Read the model definition and answer for the solid it produces. Units are mm, in the model's axes. Face numbers are marked on the shaded views. A direction names the side the tool comes from. Coordinates: 2 decimals unless noted, no trailing zeros. Write each loop counter-clockwise with the first axis right and the second up, starting at its lowest first coordinate (ties: lowest second). Pieces come first, ordered by that corner, then holes. Notation, with made-up numbers: (68, 49) -> (104, 49) arc R13 cw to (104, 54) -> close; hole circle Ø10 at (25.25, 27). An arc over 180 degrees is marked (long way). One line per item, written item: value. Start each with the question number.
from build123d import *

# Parameters (mm, degrees)
ESQUISSE1_R             = 9
ESQUISSE1_R_2           = 5.25
BOSS_EXTRU_1_DEPTH      = 13
ENL_V_MAT_EXTRU_1_DEPTH = 7
CHANFREIN1_SIZE         = 1


with BuildPart() as part:
    # Esquisse1 → Boss.-Extru.1 (new body)
    with BuildSketch(Plane.XY):
        with Locations(Location((0, 0, 0), (0, 0, 180))):
            Circle(ESQUISSE1_R)
        with Locations(Location((0, 0, 0), (0, 0, 180))):
            Circle(ESQUISSE1_R_2, mode=Mode.SUBTRACT)
    extrude(amount=BOSS_EXTRU_1_DEPTH)

    # Esquisse2 → Enlèv. mat.-Extru.1 (cut)
    with BuildSketch(Plane.XY.offset(13)):
        Polygon((3.75277675, 6.5), (-3.75277675, 6.5), (-7.505553499, 0), (-3.75277675, -6.5), (3.75277675, -6.5), (7.505553499, 0), align=None)
    extrude(amount=-ENL_V_MAT_EXTRU_1_DEPTH, mode=Mode.SUBTRACT)

    # Chanfrein1
    chanfrein1_edges = [part.edges().sort_by_distance(p)[0] for p in [
        (9, 0, 13),
    ]]
    chamfer(chanfrein1_edges, length=CHANFREIN1_SIZE)


solid = part.part
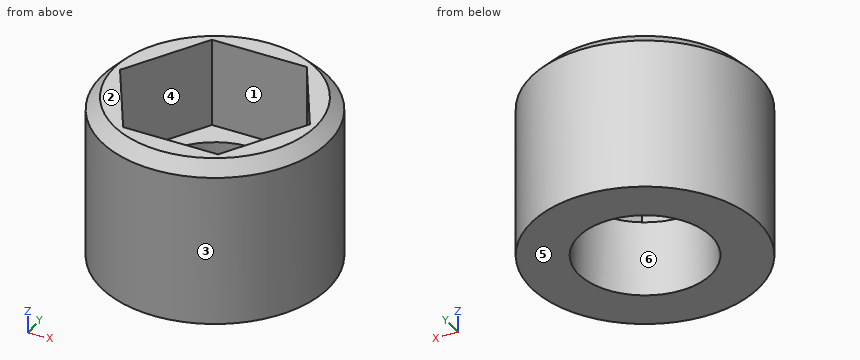
1. A tool of negligible diameter and unlimited length cuts with its end or side. For the marked faces 1 and 2, from which of +Z, -Z, +X, -X, +Y, -Y can it reach the whole face along a straight path? Write none if from no direction.
2. A cutting plane is placed at B-B on x = 0. Give the vertices of the cut face in (y, z), then the cut area to 3 significant figures.
3. For a pull along X with two mould halves and no side action, classify the marked faces 3, 4, 5 and 6 as +X half, -X half, draft (parallel to the pull), parting line (faces both ways), or undercut.
4. Find the intervals of material crossed by probe 1 along Y at (x, z) = (0, 3.7); probe 2 along Y at (x, z) = (6.25, 8.5); probe 3 along Z at (x, y) = (0.75, -6), in increasing order. Write a range as from..to.
5. Given pin 1 (2 mm diameter, centred on x = 6, z = 5, fed in from -Y); pin 2 (3 mm diameter, centred on y = -3, z = 9, fed in from +X); pin 3 (2 mm diameter, centred on x = -6.5, z = 8.5, fed in from +Y), each flat-ended and moving along its own axis, determine where each tip first touches the part or whether it passes through.
6. A cutting plane is placed at A-A on z = 7. Give the vertices of the cut face in (x, y), then the cut area to 3 significant figures.
7. A cutting plane is placed at C-C on z = 4.25. Give the vertices of the cut face in (x, y).
Derived:
1. face 1: +Z
1. face 2: +Z, +X, -X, +Y, -Y
2. outline: (-9, 0) -> (-5.25, 0) -> (-5.25, 6) -> (-6.5, 6) -> (-6.5, 13) -> (-8, 13) -> (-9, 12) -> close; (5.25, 0) -> (9, 0) -> (9, 12) -> (8, 13) -> (6.5, 13) -> (6.5, 6) -> (5.25, 6) -> close
2. area: 79.0 mm2
3. face 3: parting line
3. face 4: undercut
3. face 5: draft
3. face 6: undercut
4. probe 1: y = -9..-5.25, 5.25..9
4. probe 2: y = -6.48..-2.17, 2.17..6.48
4. probe 3: z = 0..6
5. pin 1: stops at y = -7.48
5. pin 2: stops at x = 8.87
5. pin 3: stops at y = 7.12
6. outline: circle Ø18 at (0, 0); hole (-7.51, 0) -> (-3.75, -6.5) -> (3.75, -6.5) -> (7.51, 0) -> (3.75, 6.5) -> (-3.75, 6.5) -> close
6. area: 108 mm2
7. outline: circle Ø18 at (0, 0); hole circle Ø10.5 at (0, 0)
